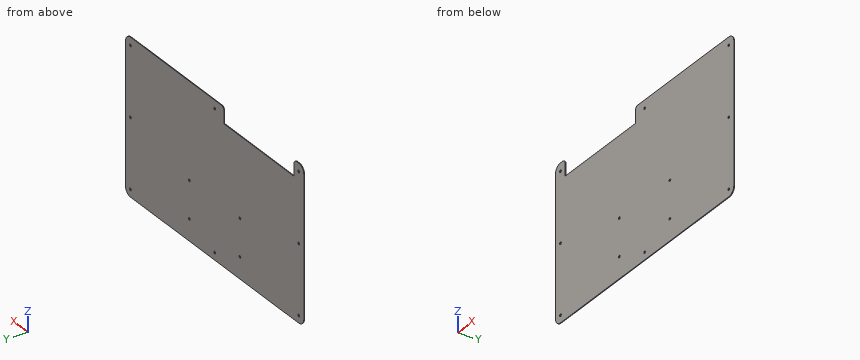
```python
from build123d import *

# Parameters (mm, degrees)
BOSS_EXTRUDE1_DEPTH           = 1
FILLET1_R                     = 10
M3_CLEARANCE_HOLE1_AT_2_COUNT = 2
M3_CLEARANCE_HOLE1_AT_2_PITCH = 95
M3_CLEARANCE_HOLE1_AT_3_COUNT = 2
M3_CLEARANCE_HOLE1_AT_3_PITCH = 95
M3_CLEARANCE_HOLE1_AT_4_COUNT = 2
M3_CLEARANCE_HOLE1_AT_4_PITCH = 193.988783761
M3_CLEARANCE_HOLE1_AT_5_COUNT = 2
M3_CLEARANCE_HOLE1_AT_5_PITCH = 351.356788607
M3_CLEARANCE_HOLE1_AT_6_COUNT = 2
M3_CLEARANCE_HOLE1_AT_6_PITCH = 338.27
M3_CLEARANCE_HOLE1_AT_7_COUNT = 2
M3_CLEARANCE_HOLE1_AT_7_PITCH = 351.356788607
M3_CLEARANCE_HOLE1_AT_8_COUNT = 2
M3_CLEARANCE_HOLE1_AT_8_PITCH = 193.988783761
M3_CLEARANCE_HOLE3_AT_2_COUNT = 2
M3_CLEARANCE_HOLE3_AT_2_PITCH = 50.8
M3_CLEARANCE_HOLE3_AT_3_COUNT = 2
M3_CLEARANCE_HOLE3_AT_3_PITCH = 101.6
M3_CLEARANCE_HOLE3_AT_4_COUNT = 2
M3_CLEARANCE_HOLE3_AT_4_PITCH = 113.592253257
FILLET2_R                     = 5


with BuildPart() as part:
    # Sketch1 → Boss-Extrude1 (new body)
    with BuildSketch(Plane(origin=(0, 0, 0), x_dir=(1, 0, 0), z_dir=(0, 1, 0))):
        Polygon((-159.635, -105.525), (-159.635, -83.525), (-18.635, -83.525), (-18.635, -105.525), (179.135, -105.525), (179.135, 105.525), (-179.135, 105.525), (-179.135, -105.525), align=None)
    extrude(amount=BOSS_EXTRUDE1_DEPTH)

    # Fillet1
    fillet1_edges = [part.edges().sort_by_distance(p)[0] for p in [
        (-179.135, 0.5, 105.525),
        (-179.135, 0.5, -105.525),
        (179.135, 0.5, -105.525),
        (179.135, 0.5, 105.525),
    ]]
    fillet(fillet1_edges, radius=FILLET1_R)

    # Sketch3 → M3 Clearance Hole1 (revolve, cut)
    with BuildSketch(Plane(origin=(169.135, 1, -0.525), x_dir=(0, 0, 1), z_dir=(1, 0, 0))):
        Polygon((0, 0), (0, 1), (1.7, 1), (1.7, 0.025), (1.725, 0), align=None)
    m3_clearance_hole1 = revolve(axis=Axis((169.135, 7.35, -0.525), (0, -1, 0)), mode=Mode.SUBTRACT)

    # M3 Clearance Hole1 at 2: M3 Clearance Hole1 ×2
    with Locations(*[(0, 0, i * M3_CLEARANCE_HOLE1_AT_2_PITCH) for i in range(1, M3_CLEARANCE_HOLE1_AT_2_COUNT)]):
        add(m3_clearance_hole1, mode=Mode.SUBTRACT)

    # M3 Clearance Hole1 at 3: M3 Clearance Hole1 ×2
    with Locations(*[(0, 0, -i * M3_CLEARANCE_HOLE1_AT_3_PITCH) for i in range(1, M3_CLEARANCE_HOLE1_AT_3_COUNT)]):
        add(m3_clearance_hole1, mode=Mode.SUBTRACT)

    # M3 Clearance Hole1 at 4: M3 Clearance Hole1 ×2
    with Locations(*[Vector(-0.871880305, 0, -0.489719035) * (i * M3_CLEARANCE_HOLE1_AT_4_PITCH) for i in range(1, M3_CLEARANCE_HOLE1_AT_4_COUNT)]):
        add(m3_clearance_hole1, mode=Mode.SUBTRACT)

    # M3 Clearance Hole1 at 5: M3 Clearance Hole1 ×2
    with Locations(*[Vector(-0.962753563, 0, -0.270380431) * (i * M3_CLEARANCE_HOLE1_AT_5_PITCH) for i in range(1, M3_CLEARANCE_HOLE1_AT_5_COUNT)]):
        add(m3_clearance_hole1, mode=Mode.SUBTRACT)

    # M3 Clearance Hole1 at 6: M3 Clearance Hole1 ×2
    with Locations(*[(-i * M3_CLEARANCE_HOLE1_AT_6_PITCH, 0, 0) for i in range(1, M3_CLEARANCE_HOLE1_AT_6_COUNT)]):
        add(m3_clearance_hole1, mode=Mode.SUBTRACT)

    # M3 Clearance Hole1 at 7: M3 Clearance Hole1 ×2
    with Locations(*[Vector(-0.962753563, 0, 0.270380431) * (i * M3_CLEARANCE_HOLE1_AT_7_PITCH) for i in range(1, M3_CLEARANCE_HOLE1_AT_7_COUNT)]):
        add(m3_clearance_hole1, mode=Mode.SUBTRACT)

    # M3 Clearance Hole1 at 8: M3 Clearance Hole1 ×2
    with Locations(*[Vector(-0.871880305, 0, 0.489719035) * (i * M3_CLEARANCE_HOLE1_AT_8_PITCH) for i in range(1, M3_CLEARANCE_HOLE1_AT_8_COUNT)]):
        add(m3_clearance_hole1, mode=Mode.SUBTRACT)

    # Sketch5 → M3 Clearance Hole3 (revolve, cut)
    with BuildSketch(Plane(origin=(50.8, 1, -25.4), x_dir=(0, 0, 1), z_dir=(1, 0, 0))):
        Polygon((0, 0), (0, 1), (1.7, 1), (1.7, 0.025), (1.725, 0), align=None)
    m3_clearance_hole3 = revolve(axis=Axis((50.8, 7.35, -25.4), (0, -1, 0)), mode=Mode.SUBTRACT)

    # M3 Clearance Hole3 at 2: M3 Clearance Hole3 ×2
    with Locations(*[(0, 0, -i * M3_CLEARANCE_HOLE3_AT_2_PITCH) for i in range(1, M3_CLEARANCE_HOLE3_AT_2_COUNT)]):
        add(m3_clearance_hole3, mode=Mode.SUBTRACT)

    # M3 Clearance Hole3 at 3: M3 Clearance Hole3 ×2
    with Locations(*[(-i * M3_CLEARANCE_HOLE3_AT_3_PITCH, 0, 0) for i in range(1, M3_CLEARANCE_HOLE3_AT_3_COUNT)]):
        add(m3_clearance_hole3, mode=Mode.SUBTRACT)

    # M3 Clearance Hole3 at 4: M3 Clearance Hole3 ×2
    with Locations(*[Vector(-0.894427191, 0, -0.447213595) * (i * M3_CLEARANCE_HOLE3_AT_4_PITCH) for i in range(1, M3_CLEARANCE_HOLE3_AT_4_COUNT)]):
        add(m3_clearance_hole3, mode=Mode.SUBTRACT)

    # Fillet2
    fillet2_edges = [part.edges().sort_by_distance(p)[0] for p in [
        (-18.635, 0.5, 105.525),
        (-159.635, 0.5, 105.525),
    ]]
    fillet(fillet2_edges, radius=FILLET2_R)


solid = part.part
```
The listing builds one solid part. Answer for the finished solid, in the listing's coordinates (mm). Give positions to 0.01 mm unless a question says otherwise; leave off trailing zeros. Write each loop counter-clockwise with the first axis right and the second up, starting at its lowest first coordinate (ties: lowest second). Pieces come first, ordered by that corner, then holes. Notation, with made-up numbers: (38, 33.5) -> (76, 33.5) arc R36 cw to (76, 67.5) -> close; hole circle Ø8 at (28.5, 54). An arc over 180 degrees is marked (long way). Use one line per item in the form item = value.
1) Straight lines are drawn through the part: probe 1 along X at (y, z) = (0.75, -76.2) (3 decimals); probe 2 along Z at (x, y) = (50.8, 0.5) (3 decimals); probe 3 along Z at (x, y) = (-108.5, 0.6) (3 decimals). For each, find the intervals that lie inside material, in ascending order.
Result:
probe_1 = -179.135 to -52.5, -49.1 to 49.1, 52.5 to 179.135
probe_2 = -105.525 to -77.9, -74.5 to -27.1, -23.7 to 105.525
probe_3 = -105.525 to 83.525
2) This flat-tipped pin is pushed along its axis until it touches: P1, Ø3, axis at x = -50.8, z = -25.4, coming from the -Y side. Where does it stop, or does it pass through?
Result:
P1 = through
3) Section B-B on x = -60.5 is taken. Write down the section's boundary in (y, z) (3 decimals), plus the area to 3 significant figures.
Result:
outline = (0, -105.525) -> (1, -105.525) -> (1, 83.525) -> (0, 83.525) -> close
area = 189 mm²
4) Section A-A on y = 0.7 is taken. Count the separate pieces of the cut face and the enclosed holes in it, plus the area to 3 significant figures.
Result:
separate_pieces = 1
enclosed_holes = 12
area = 72,300 mm²
